```python
from build123d import *

# Parameters (mm, degrees)
SKETCH1_W           = 140
SKETCH1_H           = 90
PLAIN_BOARD_DEPTH   = 3
SKETCH2_W           = 11
SKETCH2_H           = 3
MOTOR_MOUNT_DEPTH   = 3
SKETCH3_R           = 1.5
CASTER_DEPTH        = 3
SKETCH4_R           = 1.5
PCBS_DEPTH          = 3
SKETCH5_W           = 10
SKETCH5_H           = 15
SKETCH5_W_2         = 15
SKETCH5_H_2         = 25
CABLE_HOLE_DEPTH    = 3
SKETCH6_R           = 1.5
SERVO_BOARD_DEPTH   = 3
SKETCH7_R           = 1.5
SENSOR_HOLES_DEPTH  = 3
SKETCH8_R           = 1.5
SERVO_BOARD_2_DEPTH = 3
FILLET1_R           = 3
FILLET3_R           = 3


with BuildPart() as part:
    # Sketch1 → Plain Board (new body)
    with BuildSketch(Plane(origin=(0, 0, 0), x_dir=(1, 0, 0), z_dir=(0, 1, 0))):
        with Locations((70, 45)):
            Rectangle(SKETCH1_W, SKETCH1_H)
    extrude(amount=PLAIN_BOARD_DEPTH)

    # Sketch2 → Motor Mount (cut)
    with BuildSketch(Plane(origin=(0, 3, 0), x_dir=(1, 0, 0), z_dir=(0, 1, 0))):
        with Locations((47, 1.5)):
            Rectangle(SKETCH2_W, SKETCH2_H)
        with Locations((47, 22.7)):
            Rectangle(SKETCH2_W, SKETCH2_H)
        with Locations((47, 67.3)):
            Rectangle(SKETCH2_W, SKETCH2_H)
        with Locations((47, 88.5)):
            Rectangle(SKETCH2_W, SKETCH2_H)
    extrude(amount=-MOTOR_MOUNT_DEPTH, mode=Mode.SUBTRACT)

    # Sketch3 → Caster (cut)
    with BuildSketch(Plane(origin=(0, 3, 0), x_dir=(1, 0, 0), z_dir=(0, 1, 0))):
        with Locations(Location((126, 60, 0), (0, 0, 270))):
            Circle(SKETCH3_R)
        with Locations(Location((113.5, 60, 0), (0, 0, 270))):
            Circle(SKETCH3_R)
        with Locations(Location((101, 60, 0), (0, 0, 270))):
            Circle(SKETCH3_R)
        with Locations(Location((88.5, 60, 0), (0, 0, 270))):
            Circle(SKETCH3_R)
        with Locations(Location((113.5, 30, 0), (0, 0, 270))):
            Circle(SKETCH3_R)
        with Locations(Location((101, 30, 0), (0, 0, 270))):
            Circle(SKETCH3_R)
        with Locations(Location((88.5, 30, 0), (0, 0, 270))):
            Circle(SKETCH3_R)
        with Locations(Location((126, 30, 0), (0, 0, 270))):
            Circle(SKETCH3_R)
    extrude(amount=-CASTER_DEPTH, mode=Mode.SUBTRACT)

    # Sketch4 → PCBs (cut)
    with BuildSketch(Plane(origin=(0, 3, 0), x_dir=(1, 0, 0), z_dir=(0, 1, 0))):
        with Locations(Location((5, 8.9, 0), (0, 0, 270))):
            Circle(SKETCH4_R)
        with Locations(Location((26, 36, 0), (0, 0, 270))):
            Circle(SKETCH4_R)
        with Locations(Location((39, 36, 0), (0, 0, 270))):
            Circle(SKETCH4_R)
        with Locations(Location((5, 81.1, 0), (0, 0, 90))):
            Circle(SKETCH4_R)
        with Locations(Location((39, 54, 0), (0, 0, 90))):
            Circle(SKETCH4_R)
        with Locations(Location((26, 54, 0), (0, 0, 90))):
            Circle(SKETCH4_R)
    extrude(amount=-PCBS_DEPTH, mode=Mode.SUBTRACT)

    # Sketch5 → Cable Hole (cut)
    with BuildSketch(Plane(origin=(0, 3, 0), x_dir=(1, 0, 0), z_dir=(0, 1, 0))):
        with Locations((72, 45)):
            Rectangle(SKETCH5_W, SKETCH5_H)
        with Locations((59.5, 45)):
            Rectangle(SKETCH5_W_2, SKETCH5_H_2)
    extrude(amount=-CABLE_HOLE_DEPTH, mode=Mode.SUBTRACT)

    # Sketch6 → Servo Board (cut)
    with BuildSketch(Plane(origin=(0, 3, 0), x_dir=(1, 0, 0), z_dir=(0, 1, 0))):
        with Locations(Location((134, 15, 0), (0, 0, 270))):
            Circle(SKETCH6_R)
        with Locations(Location((119, 15, 0), (0, 0, 270))):
            Circle(SKETCH6_R)
        with Locations(Location((104, 15, 0), (0, 0, 270))):
            Circle(SKETCH6_R)
        with Locations(Location((89, 15, 0), (0, 0, 270))):
            Circle(SKETCH6_R)
        with Locations(Location((119, 75, 0), (0, 0, 270))):
            Circle(SKETCH6_R)
        with Locations(Location((104, 75, 0), (0, 0, 270))):
            Circle(SKETCH6_R)
        with Locations(Location((89, 75, 0), (0, 0, 270))):
            Circle(SKETCH6_R)
        with Locations(Location((134, 75, 0), (0, 0, 270))):
            Circle(SKETCH6_R)
    extrude(amount=-SERVO_BOARD_DEPTH, mode=Mode.SUBTRACT)

    # Sketch7 → Sensor Holes (cut)
    with BuildSketch(Plane(origin=(0, 3, 0), x_dir=(1, 0, 0), z_dir=(0, 1, 0))):
        with Locations(Location((134, 45, 0), (0, 0, 270))):
            Circle(SKETCH7_R)
        with Locations(Location((134, 6, 0), (0, 0, 270))):
            Circle(SKETCH7_R)
        with Locations(Location((119, 6, 0), (0, 0, 270))):
            Circle(SKETCH7_R)
        with Locations(Location((104, 6, 0), (0, 0, 270))):
            Circle(SKETCH7_R)
        with Locations(Location((89, 6, 0), (0, 0, 270))):
            Circle(SKETCH7_R)
        with Locations(Location((134, 60, 0), (0, 0, 270))):
            Circle(SKETCH7_R)
        with Locations(Location((134, 30, 0), (0, 0, 90))):
            Circle(SKETCH7_R)
        with Locations(Location((6, 45, 0), (0, 0, 270))):
            Circle(SKETCH7_R)
        with Locations(Location((6, 35, 0), (0, 0, 270))):
            Circle(SKETCH7_R)
        with Locations(Location((6, 25, 0), (0, 0, 270))):
            Circle(SKETCH7_R)
        with Locations(Location((6, 15, 0), (0, 0, 270))):
            Circle(SKETCH7_R)
        with Locations(Location((89, 84, 0), (0, 0, 90))):
            Circle(SKETCH7_R)
        with Locations(Location((104, 84, 0), (0, 0, 90))):
            Circle(SKETCH7_R)
        with Locations(Location((119, 84, 0), (0, 0, 90))):
            Circle(SKETCH7_R)
        with Locations(Location((134, 84, 0), (0, 0, 90))):
            Circle(SKETCH7_R)
        with Locations(Location((6, 75, 0), (0, 0, 90))):
            Circle(SKETCH7_R)
        with Locations(Location((6, 65, 0), (0, 0, 90))):
            Circle(SKETCH7_R)
        with Locations(Location((6, 55, 0), (0, 0, 90))):
            Circle(SKETCH7_R)
    extrude(amount=-SENSOR_HOLES_DEPTH, mode=Mode.SUBTRACT)

    # Sketch8 → Servo Board(2) (cut)
    with BuildSketch(Plane(origin=(0, 3, 0), x_dir=(1, 0, 0), z_dir=(0, 1, 0))):
        with Locations(Location((74, 60, 0), (0, 0, 270))):
            Circle(SKETCH8_R)
        with Locations(Location((74, 75, 0), (0, 0, 270))):
            Circle(SKETCH8_R)
        with Locations(Location((74, 15, 0), (0, 0, 90))):
            Circle(SKETCH8_R)
        with Locations(Location((74, 30, 0), (0, 0, 90))):
            Circle(SKETCH8_R)
    extrude(amount=-SERVO_BOARD_2_DEPTH, mode=Mode.SUBTRACT)

    # Fillet1
    fillet1_edges = [part.edges().sort_by_distance(p)[0] for p in [
        (77, 1.5, -52.5),
        (77, 1.5, -37.5),
        (67, 1.5, -37.5),
        (52, 1.5, -32.5),
        (52, 1.5, -57.5),
        (67, 1.5, -52.5),
        (0, 1.5, -90),
    ]]
    fillet(fillet1_edges, radius=FILLET1_R)

    # Fillet3
    fillet3_edges = [part.edges().sort_by_distance(p)[0] for p in [
        (140, 1.5, -90),
        (140, 1.5, 0),
        (0, 1.5, 0),
        (67, 1.5, -57.5),
        (67, 1.5, -32.5),
    ]]
    fillet(fillet3_edges, radius=FILLET3_R)


solid = part.part
```
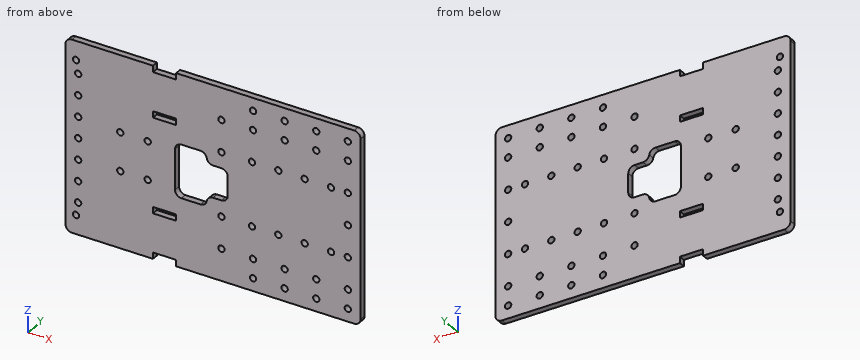
Part model, mm, in its own coordinate system. Coordinates: 2 decimals unless noted, no trailing zeros. Order: outer loops, then holes, each group sorted by start corner. A loop starts at its lowest first (then second) coordinate and runs counter-clockwise, first axis right, second up. Notation, with made-up numbers: (-8, -21) - (24, -21) arc R7 cw to (24, -17) - close; hole circle Ø4 at (7, 42). An arc over 180 degrees is marked (long way). Return JSON: item names as keys, results as strings. Group by question number.
Item 1: Cut at A-A (z = -60). List the corners of the cut face in (x, y), plus the area to 3 significant figures.
Item 2: Cut at B-B (x = 126). List the corners of the cut face in (y, z).
Item 3: Drill centre lines: probe 1 along Z at (x, y) = (113.5, 1.5); probe 2 along Z at (x, y) = (74, 1.85); probe 3 along X at (y, z) = (1.1, -84). Where is each one in solid material? Low to high. Write a range as from..to.
Item 4: Cut at C-C (y = 1.9). State how many separate pieces and enclosed holes the cut face has, plus the area to 3 significant figures.
Check values:
{
 "1": {"outline": "(0, 0) - (72.5, 0) - (72.5, 3) - (0, 3) - close; (75.5, 0) - (87, 0) - (87, 3) - (75.5, 3) - close; (90, 0) - (99.5, 0) - (99.5, 3) - (90, 3) - close; (102.5, 0) - (112, 0) - (112, 3) - (102.5, 3) - close; (115, 0) - (124.5, 0) - (124.5, 3) - (115, 3) - close; (127.5, 0) - (132.5, 0) - (132.5, 3) - (127.5, 3) - close; (135.5, 0) - (140, 0) - (140, 3) - (135.5, 3) - close", "area": "366 mm2"},
 "2": {"outline": "(0, -90) - (3, -90) - (3, -61.5) - (0, -61.5) - close; (0, -58.5) - (3, -58.5) - (3, -31.5) - (0, -31.5) - close; (0, -28.5) - (3, -28.5) - (3, 0) - (0, 0) - close"},
 "3": {"probe 1": "z = -90..-61.5, -58.5..-31.5, -28.5..0", "probe 2": "z = -90..-76.5, -73.5..-61.5, -58.5..-52.5, -37.5..-31.5, -28.5..-16.5, -13.5..0", "probe 3": "x = 0..87.5, 90.5..102.5, 105.5..117.5, 120.5..132.5, 135.5..140"},
 "4": {"separate pieces": "1", "enclosed holes": "47", "area": "11,600 mm2"}
}
